Could you check a few things on this model? Use its own coordinates, in mm. Coordinates: 2 decimals unless noted, no trailing zeros. Loops run counter-clockwise (first coordinate to the right, second up) from the corner with the lowest first, then second, coordinate; pieces in that order, holes last. Notation, with made-up numbers: M 1,47 L 59,47 A20 ccw 59,59 Z; hole C 23.25,50 d5. An arc over 180 degrees is marked long. Return JSON: item names as keys, results as strings. Group by question number.
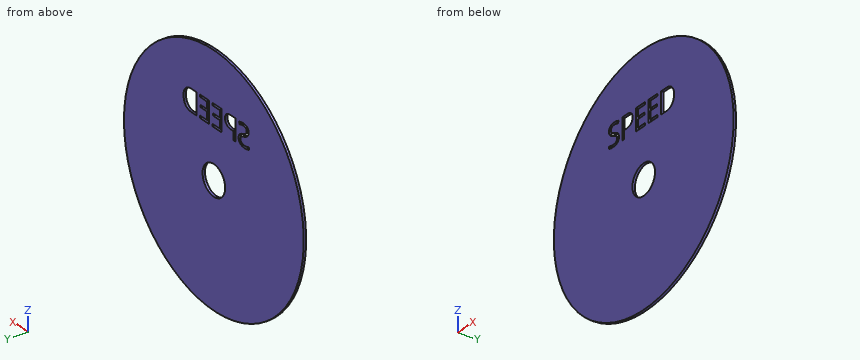
from build123d import *

# Parameters (mm, degrees)
F0_R     = 59.69
F0_R_2   = 7.493
F1_DEPTH = 0.5969


with BuildPart() as f1:
    # F0 (on Front) → F1 (new body, symmetric)
    with BuildSketch(Plane.XZ):
        Circle(F0_R)
        with BuildLine():
            add(Edge.make_bspline(
                [(-17.0897103089, 29.0026352959), (-16.4548764224, 28.3113717305), (-16.4548764224, 27.2109929938)],
                knots=[0, 0, 0, 1, 1, 1], degree=2))
            add(Edge.make_bspline(
                [(-16.4548764224, 27.2109929938), (-16.4548764224, 25.7931973138), (-17.4835424423, 24.9984793372)],
                knots=[0, 0, 0, 1, 1, 1], degree=2))
            add(Edge.make_bspline(
                [(-17.4835424423, 24.9984793372), (-18.5122084622, 24.2037613607), (-20.2756359249, 24.2037613607)],
                knots=[0, 0, 0, 1, 1, 1], degree=2))
            add(Edge.make_bspline(
                [(-20.2756359249, 24.2037613607), (-22.1848400579, 24.2037613607), (-23.2146816961, 24.6975210503)],
                knots=[0, 0, 0, 1, 1, 1], degree=2))
            Line((-23.2146816961, 24.6975210503), (-23.2146816961, 25.9013541981))
            add(Edge.make_bspline(
                [(-23.2146816961, 25.9013541981), (-22.5516329701, 25.6239082773), (-21.7733736499, 25.4616729508)],
                knots=[0, 0, 0, 1, 1, 1], degree=2))
            add(Edge.make_bspline(
                [(-21.7733736499, 25.4616729508), (-20.9951143297, 25.2994376242), (-20.2309624292, 25.2994376242)],
                knots=[0, 0, 0, 1, 1, 1], degree=2))
            add(Edge.make_bspline(
                [(-20.2309624292, 25.2994376242), (-18.9824557856, 25.2994376242), (-18.3499731356, 25.7732118025)],
                knots=[0, 0, 0, 1, 1, 1], degree=2))
            add(Edge.make_bspline(
                [(-18.3499731356, 25.7732118025), (-17.7174904857, 26.2469859808), (-17.7174904857, 27.0934311629)],
                knots=[0, 0, 0, 1, 1, 1], degree=2))
            add(Edge.make_bspline(
                [(-17.7174904857, 27.0934311629), (-17.7174904857, 27.6506742412), (-17.9420335826, 28.0068865886)],
                knots=[0, 0, 0, 1, 1, 1], degree=2))
            add(Edge.make_bspline(
                [(-17.9420335826, 28.0068865886), (-18.1665766795, 28.3630989361), (-18.6920780634, 28.6652328414)],
                knots=[0, 0, 0, 1, 1, 1], degree=2))
            add(Edge.make_bspline(
                [(-18.6920780634, 28.6652328414), (-19.2175794473, 28.9673667467), (-20.2897433446, 29.3482670786)],
                knots=[0, 0, 0, 1, 1, 1], degree=2))
            add(Edge.make_bspline(
                [(-20.2897433446, 29.3482670786), (-21.7874810696, 29.8843490273), (-22.4305442844, 30.6191104701)],
                knots=[0, 0, 0, 1, 1, 1], degree=2))
            add(Edge.make_bspline(
                [(-22.4305442844, 30.6191104701), (-23.0736074991, 31.3538719129), (-23.0736074991, 32.5365439312)],
                knots=[0, 0, 0, 1, 1, 1], degree=2))
            add(Edge.make_bspline(
                [(-23.0736074991, 32.5365439312), (-23.0736074991, 33.777996865), (-22.1413421805, 34.5127583078)],
                knots=[0, 0, 0, 1, 1, 1], degree=2))
            add(Edge.make_bspline(
                [(-22.1413421805, 34.5127583078), (-21.2090768619, 35.2475197506), (-19.6713681144, 35.2475197506)],
                knots=[0, 0, 0, 1, 1, 1], degree=2))
            add(Edge.make_bspline(
                [(-19.6713681144, 35.2475197506), (-18.0701759782, 35.2475197506), (-16.7252686333, 34.6597105963)],
                knots=[0, 0, 0, 1, 1, 1], degree=2))
            Line((-16.7252686333, 34.6597105963), (-17.1155739117, 33.5734392793))
            add(Edge.make_bspline(
                [(-17.1155739117, 33.5734392793), (-18.4463738369, 34.1306823575), (-19.7019341904, 34.1306823575)],
                knots=[0, 0, 0, 1, 1, 1], degree=2))
            add(Edge.make_bspline(
                [(-19.7019341904, 34.1306823575), (-20.6941560427, 34.1306823575), (-21.2525747393, 33.7051085298)],
                knots=[0, 0, 0, 1, 1, 1], degree=2))
            add(Edge.make_bspline(
                [(-21.2525747393, 33.7051085298), (-21.8109934358, 33.2795347022), (-21.8109934358, 32.5224365115)],
                knots=[0, 0, 0, 1, 1, 1], degree=2))
            add(Edge.make_bspline(
                [(-21.8109934358, 32.5224365115), (-21.8109934358, 31.9651934333), (-21.6052602318, 31.6078054675)],
                knots=[0, 0, 0, 1, 1, 1], degree=2))
            add(Edge.make_bspline(
                [(-21.6052602318, 31.6078054675), (-21.3995270278, 31.2504175017), (-20.9104698115, 30.9529860697)],
                knots=[0, 0, 0, 1, 1, 1], degree=2))
            add(Edge.make_bspline(
                [(-20.9104698115, 30.9529860697), (-20.4214125952, 30.6555546376), (-19.4150833231, 30.2958154352)],
                knots=[0, 0, 0, 1, 1, 1], degree=2))
            add(Edge.make_bspline(
                [(-19.4150833231, 30.2958154352), (-17.7245441955, 29.6938988613), (-17.0897103089, 29.0026352959)],
                knots=[0, 0, 0, 1, 1, 1], degree=2))
        make_face(mode=Mode.SUBTRACT)
        with BuildLine():
            add(Edge.make_bspline(
                [(-11.4702547944, 35.0946893705), (-7.4449377062, 35.0946893705), (-7.4449377062, 31.9651934333)],
                knots=[0, 0, 0, 1, 1, 1], degree=2))
            add(Edge.make_bspline(
                [(-7.4449377062, 31.9651934333), (-7.4449377062, 30.3334352211), (-8.5582482443, 29.4552483447)],
                knots=[0, 0, 0, 1, 1, 1], degree=2))
            add(Edge.make_bspline(
                [(-8.5582482443, 29.4552483447), (-9.6715587824, 28.5770614682), (-11.742998242, 28.5770614682)],
                knots=[0, 0, 0, 1, 1, 1], degree=2))
            Line((-11.742998242, 28.5770614682), (-13.0079635419, 28.5770614682))
            Line((-13.0079635419, 28.5770614682), (-13.0079635419, 24.3518892676))
            Line((-13.0079635419, 24.3518892676), (-14.2564701855, 24.3518892676))
            Line((-14.2564701855, 24.3518892676), (-14.2564701855, 35.0946893705))
            Line((-14.2564701855, 35.0946893705), (-11.4702547944, 35.0946893705))
        make_face(mode=Mode.SUBTRACT)
        Polygon((0.791444163, 25.4687266606), (0.791444163, 24.3518892676), (-5.1971555004, 24.3518892676), (-5.1971555004, 35.0946893705), (0.791444163, 35.0946893705), (0.791444163, 33.9849056872), (-3.9486488567, 33.9849056872), (-3.9486488567, 30.5238853871), (0.5045932958, 30.5238853871), (0.5045932958, 29.4211554137), (-3.9486488567, 29.4211554137), (-3.9486488567, 25.4687266606), align=None, mode=Mode.SUBTRACT)
        Circle(F0_R_2, mode=Mode.SUBTRACT)
        Polygon((9.1594952828, 25.4687266606), (9.1594952828, 24.3518892676), (3.1708956194, 24.3518892676), (3.1708956194, 35.0946893705), (9.1594952828, 35.0946893705), (9.1594952828, 33.9849056872), (4.419402263, 33.9849056872), (4.419402263, 30.5238853871), (8.8726444155, 30.5238853871), (8.8726444155, 29.4211554137), (4.419402263, 29.4211554137), (4.419402263, 25.4687266606), align=None, mode=Mode.SUBTRACT)
        with BuildLine():
            add(Edge.make_bspline(
                [(18.7255014589, 33.7062841481), (20.1139066812, 32.3178789258), (20.1139066812, 29.8255681118)],
                knots=[0, 0, 0, 1, 1, 1], degree=2))
            add(Edge.make_bspline(
                [(20.1139066812, 29.8255681118), (20.1139066812, 27.1663194981), (18.6702473984, 25.7591043828)],
                knots=[0, 0, 0, 1, 1, 1], degree=2))
            add(Edge.make_bspline(
                [(18.6702473984, 25.7591043828), (17.2265881156, 24.3518892676), (14.5156122962, 24.3518892676)],
                knots=[0, 0, 0, 1, 1, 1], degree=2))
            Line((14.5156122962, 24.3518892676), (11.5389467392, 24.3518892676))
            Line((11.5389467392, 24.3518892676), (11.5389467392, 35.0946893705))
            Line((11.5389467392, 35.0946893705), (14.8306780029, 35.0946893705))
            add(Edge.make_bspline(
                [(14.8306780029, 35.0946893705), (17.3370962366, 35.0946893705), (18.7255014589, 33.7062841481)],
                knots=[0, 0, 0, 1, 1, 1], degree=2))
        make_face(mode=Mode.SUBTRACT)
    extrude(amount=F1_DEPTH, both=True)


solid = f1.part
(1) If I drill on L1, parallel to Z at x = 0, y = -0.25; L2, parallel to Z at x = -21, y = -0.2; L3, parallel to Z at x = -1, y = 0.1, over which ranges is the centre line in solid material (lowest first)? Write a range as [from, to].
(2) Imagine slicing it at A-A, the plane z = 0. Write out the boundary of the cut face in (x, y), then the cut area to 3 significant figures.
(3) Imagine slicing it at B-B, the plane y = 0.25. Count the separate pieces of the cut face and the enclosed holes in it, then the cut area to 3 significant figures.
(4) Imagine slicing it at C-C, the plane x = 46. Write out the boundary of the cut face in (y, z).
(5) Imagine slicing it at D-D, the plane z = -20. Write out the boundary of the cut face in (x, y).
(6) Will these pins go through, and if not, where does the flat tip stop? P1, Ø0.6, axis at y = 0, z = 32.5, coming from the -X side; P2, Ø0.6, axis at y = 0, z = 34.5, coming from the -X side; P3, Ø12, axis at x = 0, z = 0, coming from the +Y side.
Checks:
{
 "1": {"L1": "[-59.69, -7.49], [7.49, 24.35], [25.47, 29.42], [30.52, 33.98], [35.09, 59.69]", "L2": "[-55.87, 24.22], [25.34, 29.64], [31.01, 33.86], [35.08, 55.87]", "L3": "[-59.68, -7.43], [7.43, 24.35], [25.47, 29.42], [30.52, 33.98], [35.09, 59.68]"},
 "2": {"outline": "M -59.69,-0.6 L -7.49,-0.6 L -7.49,0.6 L -59.69,0.6 Z; M 7.49,-0.6 L 59.69,-0.6 L 59.69,0.6 L 7.49,0.6 Z", "area": "125 mm²"},
 "3": {"separate pieces": "1", "enclosed holes": "6", "area": "10,800 mm²"},
 "4": {"outline": "M -0.6,-38.04 L 0.6,-38.04 L 0.6,38.04 L -0.6,38.04 Z"},
 "5": {"outline": "M -56.24,-0.6 L 56.24,-0.6 L 56.24,0.6 L -56.24,0.6 Z"},
 "6": {"P1": "x = -50.26", "P2": "x = -48.92", "P3": "through"}
}
